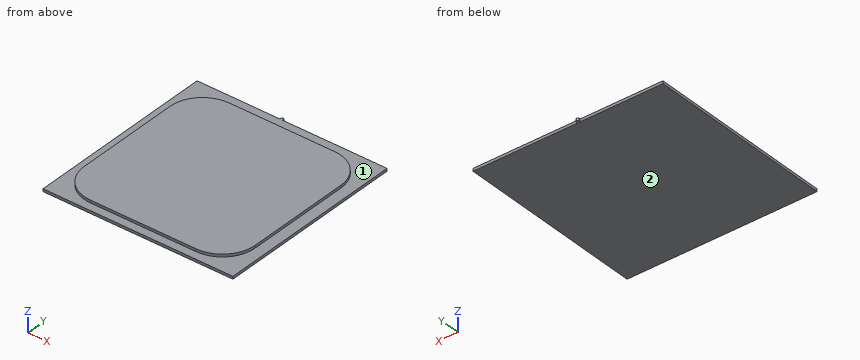
Autodesk Inventor part; units mm, degrees
ref_plane "YZ Plane" through (0, 0, 0) normal (1, 0, 0) x (0, 1, 0)
ref_plane "XZ Plane" through (0, 0, 0) normal (0, 1, 0) x (-1, 0, 0)
ref_plane "XY Plane" through (0, 0, 0) normal (0, 0, 1) x (1, 0, 0)
sketch "Sketch1" plane through (0, 0, 0) normal (0, 0, 1) x (1, 0, 0)
  line L0 (0, 0) -> (17.78, 0)
  line L1 (17.78, 0) -> (17.78, 17.78)
  line L2 (17.78, 17.78) -> (0, 17.78)
  line L3 (0, 17.78) -> (0, 0)
  dimension "d0" = 17.78
extrude "Extrusion1" add sketch "Sketch1" along normal blind 0.254
sketch "Sketch2" plane through (0, 0, 0.254) normal (0, 0, 1) x (1, 0, 0)
  line L0 (0.762, 16.764) -> (16.764, 16.764)
  line L1 (16.764, 16.764) -> (16.764, 0.762)
  line L2 (16.764, 0.762) -> (0.762, 0.762)
  line L3 (0.762, 0.762) -> (0.762, 16.764)
  line L4 (0, 0) -> (17.78, 0)
  line L5 (0, 17.78) -> (0, 0)
  point P0 (0.762, 0.762)
  dimension "d3" = 16.002
  dimension "d4" = 0.762
  dimension "d5" = 0.762
extrude "Extrusion2" add sketch "Sketch2" along normal blind 0.254
fillet "Fillet1" radius 3.048 1 edges at (0.762, 0.762, 0.381)
fillet "Fillet2" radius 3.048 3 edges at (16.764, 0.762, 0.381) (16.764, 16.764, 0.381) (0.762, 16.764, 0.381)
sketch "Sketch3" plane through (0, 17.78, 0) normal (0, 1, 0) x (1, 0, 0)
  line L0 (17.78, 0) -> (0, 0)
  line L1 (0, -0.254) -> (17.78, -0.254)
  line L2 (7.747, 0) -> (8.001, 0)
  line L3 (8.001, 0) -> (8.001, -0.254)
  line L4 (8.001, -0.254) -> (7.747, -0.254)
  line L5 (7.747, -0.254) -> (7.747, 0)
  dimension "d10" = 7.747
  dimension "d11" = 0.254
extrude "Extrusion3" add sketch "Sketch3" along normal blind 0.254
fillet "Fillet3" radius 0.127 2 edges at (8.001, 18.034, 0.127) (7.747, 18.034, 0.127)
properties part number "plate" material "Gold"
Read the model definition and answer for the solid it produces. Units are mm, in the model's axes. Face numbers are marked on the shaded views. A direction names the side the tool comes from. Round coordinates to 2 decimals unless told otherwise and drop trailing zeros. Write each loop counter-clockwise with the first axis right and the second up, starting at its lowest first coordinate (ties: lowest second). Pieces come first, ordered by that corner, then holes. Notation, with made-up numbers: M -6.5,79 L 31.5,79 A12 ccw 31.5,97 Z; hole C 65,-13 d3. An arc over 180 degrees is marked long. One line per item, written item: value.
Q1. Find section A-A on y = 9. Write down the section's boundary in (x, z).
Data:
outline: M 0,0 L 17.78,0 L 17.78,0.25 L 16.76,0.25 L 16.76,0.51 L 0.76,0.51 L 0.76,0.25 L 0,0.25 Z
Q2. Which of the six approach directions +Z, -Z, +X, -X, +Y, -Y give full straight-line access (tool end or side, diameter ignored) to the marked faces 1 and 2?
Data:
face 1: +Z
face 2: -Z, +X, -X, +Y, -Y
Q3. Straight lines are drawn through the part: line 1 (Y direction, x = 11.5, z = 0.1); line 2 (Y direction, x = 7, z = 0.3). For each, find the intervals that lie inside material, in ascending order. Write a range as [from, to].
Data:
line 1: [0, 17.78]
line 2: [0.76, 16.76]
